Verification items for the finished model (mm, model axes). A direction names the side the tool comes from. Round coordinates to 2 decimals unless told otherwise and drop trailing zeros. Write each loop counter-clockwise with the first axis right and the second up, starting at its lowest first coordinate (ties: lowest second). Pieces come first, ordered by that corner, then holes. Notation, with made-up numbers: (-8, 1) - (23, 1) arc R16 cw to (23, 18) - close; hole circle Ø2 at (4, 83.25). An arc over 180 degrees is marked (long way). Answer as a JSON object with one key per item and string values.
```python
from build123d import *

# Parameters (mm, degrees)
SKETCH1_W           = 36
SKETCH1_H           = 36
BOSS_EXTRUDE1_DEPTH = 11
SKETCH2_W           = 24
SKETCH2_H           = 24
BOSS_EXTRUDE2_DEPTH = 3
SKETCH3_R           = 6
BOSS_EXTRUDE3_DEPTH = 6
SKETCH4_R           = 7
BOSS_EXTRUDE4_DEPTH = 2.5
SKETCH5_R           = 9
BOSS_EXTRUDE5_DEPTH = 3


with BuildPart() as part:
    # Sketch1 → Boss-Extrude1 (new body)
    with BuildSketch(Plane(origin=(0, 0, 0), x_dir=(1, 0, 0), z_dir=(0, 1, 0))):
        Rectangle(SKETCH1_W, SKETCH1_H)
    extrude(amount=BOSS_EXTRUDE1_DEPTH)

    # Sketch2 → Boss-Extrude2 (add)
    with BuildSketch(Plane(origin=(0, 11, 0), x_dir=(1, 0, 0), z_dir=(0, 1, 0))):
        Rectangle(SKETCH2_W, SKETCH2_H)
    extrude(amount=BOSS_EXTRUDE2_DEPTH)

    # Sketch3 → Boss-Extrude3 (add)
    with BuildSketch(Plane(origin=(0, 14, 0), x_dir=(1, 0, 0), z_dir=(0, 1, 0))):
        with Locations(Location((0, 0, 0), (0, 0, 270))):
            Circle(SKETCH3_R)
    extrude(amount=BOSS_EXTRUDE3_DEPTH)

    # Sketch4 → Boss-Extrude4 (add)
    with BuildSketch(Plane(origin=(0, 20, 0), x_dir=(1, 0, 0), z_dir=(0, 1, 0))):
        with Locations(Location((0, 0, 0), (0, 0, 270))):
            Circle(SKETCH4_R)
    extrude(amount=BOSS_EXTRUDE4_DEPTH)

    # Sketch5 → Boss-Extrude5 (add)
    with BuildSketch(Plane(origin=(0, 22.5, 0), x_dir=(1, 0, 0), z_dir=(0, 1, 0))):
        with Locations(Location((0, 0, 0), (0, 0, 270))):
            Circle(SKETCH5_R)
    extrude(amount=BOSS_EXTRUDE5_DEPTH)


solid = part.part
```
Q1. Section check D-D, the plane y = 15. Record the cut outline in (x, z).
Geometry check:
{"outline": "circle Ø12 at (0, 0)"}
Q2. Section check C-C, the plane x = 0. Record the cut outline in (y, z), then the cut area to 3 significant figures.
Geometry check:
{"outline": "(0, -18) - (11, -18) - (11, -12) - (14, -12) - (14, -6) - (20, -6) - (20, -7) - (22.5, -7) - (22.5, -9) - (25.5, -9) - (25.5, 9) - (22.5, 9) - (22.5, 7) - (20, 7) - (20, 6) - (14, 6) - (14, 12) - (11, 12) - (11, 18) - (0, 18) - close", "area": "629 mm2"}
Q3. Release check for a two-part mould opening along Y. For faces 1 (the flat face through (-18, 5, 0)), 2 (the cylindrical face through (-6.834, 21.232, -1.517)), 3 (the flat face through (-6, 14, -3)), 4 (the flat face through (0, 25.5, 0)) record: released by +Y, released by -Y, zero draft, split by the parting line, or undercut.
Geometry check:
{"face 1": "zero draft", "face 2": "undercut", "face 3": "undercut", "face 4": "released by +Y"}
Q4. Material ranges on line 1 along Y through (x, z) = (4.5, 5); line 2 along X through (y, z) = (11.75, 1); line 3 along Y through (x, z) = (3.5, -10), recorded low to high. Write a range as [from, to].
Geometry check:
{"line 1": "y = [0, 14], [20, 25.5]", "line 2": "x = [-12, 12]", "line 3": "y = [0, 14]"}
Q5. Section check B-B, the plane z = -9.5. Record the cut outline in (x, y), then the cut area to 3 significant figures.
Geometry check:
{"outline": "(-18, 0) - (18, 0) - (18, 11) - (12, 11) - (12, 14) - (-12, 14) - (-12, 11) - (-18, 11) - close", "area": "468 mm2"}
Q6. Set-up check for faces 5 (the flat face through (-12, 12, 0)), 6 (the flat face through (2, 20, 6)), 7 (the flat face through (0, 12, 12)), 8 (the flat face through (12, 12, 0)), 9 (the cylindrical face through (2.703, 23.979, 8.584)): record each of +Z, -Z, +X, -X, +Y, -Y from which the full face is reachable in a straight line by a thin tool's end or side.
Geometry check:
{"face 5": "+Z, -Z, -X, +Y", "face 6": "none", "face 7": "+Z, +X, -X, +Y", "face 8": "+Z, -Z, +X, +Y", "face 9": "+Y"}
Q7. Section check A-A, the plane x = -11. Record the cut outline in (y, z).
Geometry check:
{"outline": "(0, -18) - (11, -18) - (11, -12) - (14, -12) - (14, 12) - (11, 12) - (11, 18) - (0, 18) - close"}
Q8. Gauge pin test, flat ends, axial feed: P1, Ø3, axis at x = -6.5, y = 14, coming from the -Z side; P2, Ø2.5, axis at x = 0.5, y = 13, coming from the +Z side; P3, Ø2.5, axis at y = 12.5, z = 3.5, coming from the -X side. Record the tip position at first contact, or that the pin passes through.
Geometry check:
{"P1": "stops at z = -12", "P2": "stops at z = 12", "P3": "stops at x = -12"}
